Input: part model. Units: mm. Frame: model coordinates. Face numbers are marked on the shaded views. Give positions to 0.01 mm unless a question says otherwise; leave off trailing zeros. Loops run counter-clockwise (first coordinate to the right, second up) from the corner with the lowest first, then second, coordinate; pieces in that order, holes last. Notation, with made-up numbers: (-11, 74) -> (44, 74) arc R10 cw to (44, 79) -> close; hole circle Ø3 at (78.5, 86). An arc over 180 degrees is marked (long way). Answer as a JSON object with one key per item and string values. Group by question number.
```python
from build123d import *

# Parameters (mm, degrees)
SKETCH1_R           = 2.2606
BOSS_EXTRUDE1_DEPTH = 25.8064
BOSS_EXTRUDE2_DEPTH = 2.9718
SKETCH3_R           = 17.5514
BOSS_EXTRUDE3_DEPTH = 5.2832
FILLET1_R           = 1.27
SKETCH4_R           = 8.4709
BOSS_EXTRUDE4_DEPTH = 4.445
FILLET2_R           = 1.27


with BuildPart() as part:
    # Sketch1 → Boss-Extrude1 (new body)
    with BuildSketch(Plane(origin=(0, 0, 0), x_dir=(0, 0, -1), z_dir=(1, 0, 0))):
        Circle(SKETCH1_R)
    extrude(amount=BOSS_EXTRUDE1_DEPTH)

    # Sketch2 → Boss-Extrude2 (add)
    with BuildSketch(Plane(origin=(7.366, 0, 0), x_dir=(0, 0, -1), z_dir=(1, 0, 0))):
        with BuildLine():
            Line((-34.4932, 5.1562), (-10.795, 5.1562))
            ThreePointArc((-10.795, 5.1562), (-4.640157933, 3.106734389), (0, -1.426622482))
            Line((0, -1.426622482), (0, 1.341450991))
            ThreePointArc((0, 1.341450991), (-16.651297211, 8.631590684), (-34.4932, 5.1562))
        make_face()
    extrude(amount=BOSS_EXTRUDE2_DEPTH)

    # Sketch3 → Boss-Extrude3 (add)
    with BuildSketch(Plane.XZ.offset(-5.1562)):
        with Locations(Location((8.8519, 28.3464, 0), (0, 0, 270))):
            Circle(SKETCH3_R)
    extrude(amount=BOSS_EXTRUDE3_DEPTH)

    # Fillet1
    fillet1_edges = [part.edges().sort_by_distance(p)[0] for p in [
        (8.8519, 5.1562, 45.8978),
        (8.8519, -0.127, 45.8978),
    ]]
    fillet(fillet1_edges, radius=FILLET1_R)

    # Sketch4 → Boss-Extrude4 (add)
    with BuildSketch(Plane(origin=(0, 5.1562, 0), x_dir=(1, 0, 0), z_dir=(0, 1, 0))):
        with Locations(Location((25.032233899, -30.157692599, 0), (0, 0, 98.691062449))):
            Circle(SKETCH4_R)
    extrude(amount=BOSS_EXTRUDE4_DEPTH)

    # Fillet2
    fillet2_edges = [part.edges().sort_by_distance(p)[0] for p in [
        (26.312242996, 9.6012, 38.531325234),
    ]]
    fillet(fillet2_edges, radius=FILLET2_R)


solid = part.part
```
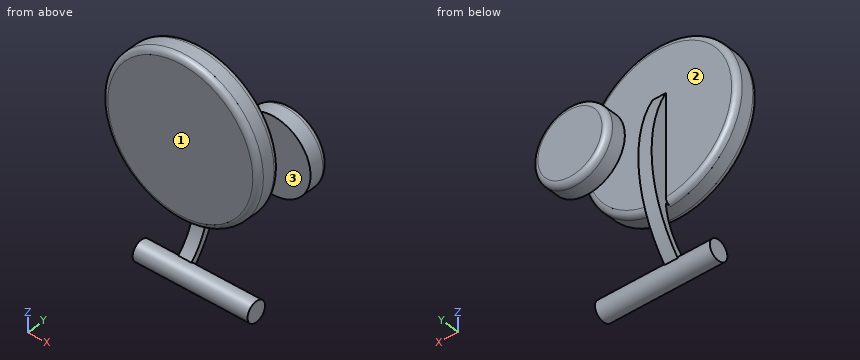
Q1. Pull-direction query (Y, two-part tool) for the marked faces 1, 2 and 3; classes: +Y half, -Y half, draft (parallel to the pull), parting line (faces both ways), or undercut.
Q2. Section C-C on z = 6.5. Return the cut outline in (x, y), then the cut area to 3 significant figures.
Q3. Section A-A on y = 3. Return the cut outline in (x, z) (3 decimals), then the cut area to 3 significant figures.
Q4. Ray query, probe 1 along Y at (x, z) = (4.5, 26); probe 2 along X at (y, z) = (1.75, 28); probe 3 along Z at (x, y) = (1, 0.5) (3 decimals). Return the intervals inside material, ascending.
Q5. Section B-B on z = 0. Return the cut outline in (x, y), then the cut area to 3 significant figures.
Q6. Pin query (flat end, axial travel): pin 1 Ø5 at (y, z) = (6, 25.5) entering from +X; pin 2 Ø1 at (y, z) = (6.5, 28) entering from +X; pin 3 Ø6 at (x, z) = (26, 32.5) entering from -Y. Return the tip coordinate at first contact, or that it passes through.
Numbers:
{
 "1": {"face 1": "-Y half", "face 2": "+Y half", "face 3": "undercut"},
 "2": {"outline": "(7.37, 4.06) -> (10.34, 4.06) -> (10.34, 5.66) -> (7.37, 5.66) -> close", "area": "4.76 mm²"},
 "3": {"outline": "circle Ø35.103 at (8.852, 28.346); (7.366, 2.087) -> (10.338, 2.087) -> (10.338, 4.468) -> (7.366, 4.468) -> close", "area": "975 mm²"},
 "4": {"probe 1": "y = -0.13 to 5.16", "probe 2": "x = -8.7 to 26.4", "probe 3": "z = -2.205 to 2.205, 12.845 to 43.848"},
 "5": {"outline": "(0, -2.26) -> (25.81, -2.26) -> (25.81, 2.26) -> (0, 2.26) -> close", "area": "117 mm²"},
 "6": {"pin 1": "stops at x = 33.22", "pin 2": "stops at x = 33.34", "pin 3": "stops at y = -0.13"}
}
